```python
from build123d import *

# Parameters (mm, degrees)
SKETCH1_R           = 1
SKETCH1_R_2         = 0.75
BOSS_EXTRUDE1_DEPTH = 90
CUT_EXTRUDE1_DEPTH  = 1


with BuildPart() as part:
    # Sketch1 → Boss-Extrude1 (new body)
    with BuildSketch(Plane(origin=(0, 0, 0), x_dir=(0, 0, -1), z_dir=(1, 0, 0))):
        with Locations(Location((0, 0, 0), (0, 0, 180))):
            Circle(SKETCH1_R)
        with Locations(Location((0, 0, 0), (0, 0, 180))):
            Circle(SKETCH1_R_2, mode=Mode.SUBTRACT)
    extrude(amount=BOSS_EXTRUDE1_DEPTH)

    # Sketch2 → Cut-Extrude1 (cut)
    with BuildSketch(Plane.ZY):
        with BuildLine():
            Line((-0.304, 0.610565492), (-0.304, 1.099202537))
            Line((-0.304, 1.099202537), (0.304, 1.099202537))
            Line((0.304, 1.099202537), (0.304, 0.610565492))
            ThreePointArc((0.304, 0.610565492), (0, 0.306565492), (-0.304, 0.610565492))
        make_face()
    extrude(amount=-CUT_EXTRUDE1_DEPTH, mode=Mode.SUBTRACT)


solid = part.part
```
Input: part model. Units: mm. Frame: model coordinates. Give positions to 0.01 mm unless a question says otherwise; leave off trailing zeros. Order: outer loops, then holes, each group sorted by start corner. A loop starts at its lowest first (then second) coordinate and runs counter-clockwise, first axis right, second up.
1. Section B-B on z = 0. Return the cut outline in (x, y).
Derived:
outline: (0, -1) - (90, -1) - (90, -0.75) - (0, -0.75) - close; (1, 0.75) - (90, 0.75) - (90, 1) - (1, 1) - close
2. Section C-C on x = 24. Return the cut outline in (y, z), and give its area (3 significant figures).
Derived:
outline: circle Ø2 at (0, 0); hole circle Ø1.5 at (0, 0)
area: 1.37 mm2
3. Mould query, pull axis Y, two halves, no side actions, for faces 1 (the cylindrical face through (44.37, -0.225, 0.715)), 2 (the cylindrical face through (44, 1, 0)). Classes: released by +Y, released by -Y, zero draft, split by the parting line, or undercut.
Derived:
face 1: undercut
face 2: split by the parting line
4. Material intervals for L1, parallel to Z at x = 51.5, y = -0.1; L2, parallel to Y at x = 42, z = 0; L3, parallel to Y at x = 24, z = -0.5, sorted ascending.
Derived:
L1: z = -0.99 to -0.74, 0.74 to 0.99
L2: y = -1 to -0.75, 0.75 to 1
L3: y = -0.87 to -0.56, 0.56 to 0.87
5. Section A-A on y = 0. Return the cut outline in (x, z).
Derived:
outline: (0, -1) - (90, -1) - (90, -0.75) - (0, -0.75) - close; (0, 0.75) - (90, 0.75) - (90, 1) - (0, 1) - close
